Could you check a few things on this model? Use its own coordinates, in mm. Face numbers are marked on the shaded views. A direction names the side the tool comes from. Coordinates: 2 decimals unless noted, no trailing zeros. Write each loop counter-clockwise with the first axis right and the second up, starting at its lowest first coordinate (ties: lowest second). Pieces come first, ordered by that corner, then holes. Notation, with made-up numbers: (-13, 59.25) - (35, 59.25) arc R22 cw to (35, 87.25) - close; hole circle Ø11 at (9, 27.5). An arc over 180 degrees is marked (long way). Answer as a JSON object with one key per item and string values. Group by question number.
1) If we section it at C-C (z = 1): Write out the boundary of the cut face in (x, y), plus the area to 3 significant figures.
2) If we section it at B-B (x = -8.5): Write out the boundary of the cut face in (y, z), plus the area to 3 significant figures.
3) If we section it at A-A (y = 9): Write out the boundary of the cut face in (x, z).
4) We'd pull the mould along X, two halves only. Please class the marked faces 4, 5 and 6: released by +X, released by -X, zero draft, split by the parting line, or undercut.
5) If we section it at D-D (z = 9): Write out the boundary of the cut face in (x, y), plus the area to 3 significant figures.
6) On a 3-axis mill with a long thin cutter (end or side, diameter ignored), from which of +Z, -Z, +X, -X, +Y, -Y can I reach the whole of each face in a straight line? I mean the marked faces 1, 2 and 3. Say none if no direction works.
7) Please list where these lines run through material, in increasing order: line 1 along X through (y, z) = (4.75, -10.5); line 2 along Z through (x, y) = (-8, 3.75); line 3 along Y through (x, z) = (-21, 2.5).
8) Will these pins go through, and if not, where does the flat tip stop? pin 1 Ø9.5 at (x, z) = (24.5, -13.5) entering from +Y; pin 2 Ø3 at (x, y) = (8, 5.5) entering from -Z; pin 3 Ø0.5 at (x, y) = (-21, 8) entering from +Z; pin 4 Ø4 at (x, z) = (-8.5, -6) entering from +Y.
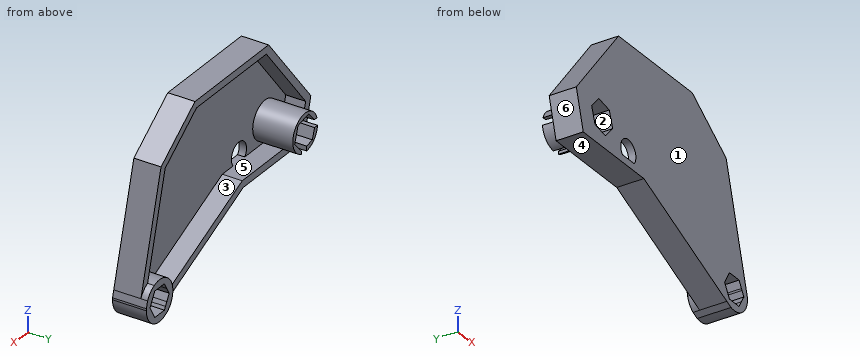
```python
from build123d import *

# Parameters (mm, degrees)
F0_R     = 3.93
F1_DEPTH = 1.5
F2_DEPTH = 5.62
F3_DEPTH = 9.8
F4_DEPTH = 7
F7_DEPTH = 3


with BuildPart() as f1:
    # F0 (on Front) → F1 (new body)
    with BuildSketch(Plane.XZ):
        with BuildLine():
            Line((-22.505389868, -2.0895681901), (-11.2077256692, -2.0895681901))
            ThreePointArc((-11.2077256692, -2.0895681901), (-9.3285928413, 1.8148319814), (-7.4494600134, -2.0895681901))
            Line((-7.4494600134, -2.0895681901), (-4.0605032691, -2.0895681901))
            Line((-4.0605032691, -2.0895681901), (20.2483866423, -12.9712812224))
            ThreePointArc((20.2483866423, -12.9712812224), (21.5778297936, -8.6925507754), (26.0093476524, -8.0317915166))
            Line((26.0093476524, -8.0317915166), (20.4338732281, 12.2993333716))
            Line((20.4338732281, 12.2993333716), (10.4662147941, 19.5698092025))
            Line((10.4662147941, 19.5698092025), (-11.712607269, 19.5698092025))
            Line((-11.712607269, 19.5698092025), (-24.1958881701, 4.0444751638))
            Line((-24.1958881701, 4.0444751638), (-22.505389868, -2.0895681901))
        make_face()
        with Locations((-17.636482101, 2.2704318099)):
            Circle(F0_R, mode=Mode.SUBTRACT)
    extrude(amount=-F1_DEPTH)

    # F0 (on Front) → F2 (join)
    with BuildSketch(Plane.XZ):
        with BuildLine():
            Line((-7.4494600134, -2.0895681901), (-9.3285928413, -2.0895681901))
            Line((-9.3285928413, -2.0895681901), (-11.2077256692, -2.0895681901))
            Line((-11.2077256692, -2.0895681901), (-22.505389868, -2.0895681901))
            Line((-22.505389868, -2.0895681901), (-24.1958881701, 4.0444751638))
            Line((-24.1958881701, 4.0444751638), (-11.712607269, 19.5698092025))
            Line((-11.712607269, 19.5698092025), (10.4662147941, 19.5698092025))
            Line((10.4662147941, 19.5698092025), (20.4338732281, 12.2993333716))
            Line((20.4338732281, 12.2993333716), (26.0093476524, -8.0317915166))
            ThreePointArc((26.0093476524, -8.0317915166), (27.2575403042, -8.8716753621), (28.1309747483, -10.096625174))
            Line((28.1309747483, -10.096625174), (21.7417066053, 13.2020214837))
            Line((21.7417066053, 13.2020214837), (10.9551470408, 21.0698092025))
            Line((10.9551470408, 21.0698092025), (-12.4312654999, 21.0698092025))
            Line((-12.4312654999, 21.0698092025), (-25.8459559813, 4.3860902027))
            Line((-25.8459559813, 4.3860902027), (-23.6479217985, -3.5895681901))
            Line((-23.6479217985, -3.5895681901), (-4.3809167168, -3.5895681901))
            Line((-4.3809167168, -3.5895681901), (21.9651791943, -15.3832229506))
            ThreePointArc((21.9651791943, -15.3832229506), (20.887904522, -14.3330472271), (20.2483866423, -12.9712812224))
            Line((20.2483866423, -12.9712812224), (-4.0605032691, -2.0895681901))
            Line((-4.0605032691, -2.0895681901), (-7.4494600134, -2.0895681901))
        make_face()
    extrude(amount=-F2_DEPTH)

    # F0 (on Front) → F3 (join)
    with BuildSketch(Plane.XZ):
        with Locations((-17.636482101, 2.2704318099)):
            Circle(F0_R)
        Polygon((-16.5711225386, -0.9650499681), (-19.9058117331, -0.2699375244), (-20.9711712955, 2.9655442536), (-18.7018416635, 5.5059135879), (-15.367152469, 4.8108011442), (-14.3017929065, 1.5753193661), align=None, mode=Mode.SUBTRACT)
    extrude(amount=-F3_DEPTH)

    # F0 (on Front) → F4 (join)
    with BuildSketch(Plane.XZ):
        with BuildLine():
            Line((22.4537352546, -13.9584908738), (20.2483866423, -12.9712812224))
            ThreePointArc((20.2483866423, -12.9712812224), (20.887904522, -14.3330472271), (21.9651791943, -15.3832229506))
            Line((21.9651791943, -15.3832229506), (23.2829635099, -15.9731203426))
            ThreePointArc((23.2829635099, -15.9731203426), (26.905846951, -15.2153095013), (28.5319774541, -11.8903641956))
            ThreePointArc((28.5319774541, -11.8903641956), (28.5271836329, -11.6894581734), (28.5128130807, -11.4890094325))
            Line((28.5128130807, -11.4890094325), (28.1309747483, -10.096625174))
            ThreePointArc((28.1309747483, -10.096625174), (27.2575403042, -8.8716753621), (26.0093476524, -8.0317915166))
            Line((26.0093476524, -8.0317915166), (26.7851210641, -10.8606711631))
            Line((26.7851210641, -10.8606711631), (27.3796146136, -11.8903641956))
            Line((27.3796146136, -11.8903641956), (26.6146255071, -13.2153641953))
            Line((26.6146255071, -13.2153641953), (25.8496364003, -14.5403641956))
            Line((25.8496364003, -14.5403641956), (24.3196581869, -14.5403641956))
            Line((24.3196581869, -14.5403641956), (22.7896799735, -14.5403641956))
            Line((22.7896799735, -14.5403641956), (22.4537352546, -13.9584908738))
        make_face()
        with BuildLine():
            ThreePointArc((26.0093476524, -8.0317915166), (21.5778297936, -8.6925507754), (20.2483866423, -12.9712812224))
            Line((20.2483866423, -12.9712812224), (22.4537352546, -13.9584908738))
            Line((22.4537352546, -13.9584908738), (22.024690908, -13.2153642668))
            Line((22.024690908, -13.2153642668), (21.2597017602, -11.8903641956))
            Line((21.2597017602, -11.8903641956), (22.0246909248, -10.5653640952))
            Line((22.0246909248, -10.5653640952), (22.7896799735, -9.2403641956))
            Line((22.7896799735, -9.2403641956), (24.3196581869, -9.2403641956))
            Line((24.3196581869, -9.2403641956), (25.8496364003, -9.2403641956))
            Line((25.8496364003, -9.2403641956), (26.6146254836, -10.5653641553))
            Line((26.6146254836, -10.5653641553), (26.7851210641, -10.8606711631))
            Line((26.7851210641, -10.8606711631), (26.0093476524, -8.0317915166))
        make_face()
    extrude(amount=-F4_DEPTH)

    # F6 (on face) → F7 (cut)
    with BuildSketch(Plane(origin=(0, 9.8, 0), x_dir=(-1, 0, 0), z_dir=(0, 1, 0))):
        with BuildLine():
            ThreePointArc((16.5027278304, -1.4924794638), (17.2955343411, -1.6447507689), (18.1027278304, -1.6318130466))
            Line((18.1027278304, -1.6318130466), (18.1027278304, -0.6457884612))
            Line((18.1027278304, -0.6457884612), (16.5711225386, -0.9650499681))
            Line((16.5711225386, -0.9650499681), (16.5027278304, -0.8884864682))
            Line((16.5027278304, -0.8884864682), (16.5027278304, -1.4924794638))
        make_face()
        with BuildLine():
            Line((20.9711712955, 2.9655442536), (20.60459144, 1.852246467))
            Line((20.60459144, 1.852246467), (21.544169527, 1.852246467))
            ThreePointArc((21.544169527, 1.852246467), (21.5608999932, 2.0610417242), (21.566482101, 2.2704318099))
            ThreePointArc((21.566482101, 2.2704318099), (21.520739578, 2.8682978924), (21.3845768325, 3.452246467))
            Line((21.3845768325, 3.452246467), (20.5363968161, 3.452246467))
            Line((20.5363968161, 3.452246467), (20.9711712955, 2.9655442536))
        make_face()
    extrude(amount=-F7_DEPTH, mode=Mode.SUBTRACT)


solid = f1.part
```
Here are the results:
{
 "1": {"outline": "(-24.91, 0) - (-20.32, 0) - (-20.32, 9.8) - (-21.36, 9.8) - (-21.36, 1.5) - (-23.36, 1.5) - (-23.36, 5.62) - (-24.91, 5.62) - close; (-14.82, 0) - (-11.13, 0) - (-11.13, 1.5) - (-13.92, 1.5) - (-13.92, 9.8) - (-14.82, 9.8) - close; (-7.52, 0) - (25.09, 0) - (25.09, 5.62) - (23.53, 5.62) - (23.53, 1.5) - (-7.52, 1.5) - close", "area": "90.2 mm²"},
 "2": {"outline": "(0, -3.59) - (5.62, -3.59) - (5.62, -2.09) - (0, -2.09) - close; (0, 1.67) - (1.5, 1.67) - (1.5, 19.57) - (5.62, 19.57) - (5.62, 21.07) - (0, 21.07) - close", "area": "43.7 mm²"},
 "3": {"outline": "(-21.54, 1.85) arc R3.93 ccw to (-18.1, -1.63) - (-18.1, -0.65) - (-19.91, -0.27) - (-20.6, 1.85) - close; (-21.38, 3.45) - (-20.54, 3.45) - (-18.7, 5.51) - (-15.37, 4.81) - (-14.3, 1.58) - (-16.5, -0.89) - (-16.5, -1.49) arc R3.93 ccw (long way) to start"},
 "4": {"face 4": "zero draft", "face 5": "undercut", "face 6": "released by -X"},
 "5": {"outline": "(-22.14, 0) - (22.89, 0) - (22.89, 5.62) - (21.34, 5.62) - (21.34, 1.5) - (-20.21, 1.5) - (-20.21, 5.62) - (-22.14, 5.62) - close", "area": "81.9 mm²"},
 "6": {"face 1": "+Z, -Z, +X, -X, -Y", "face 2": "+Y, -Y", "face 3": "+Y"},
 "7": {"line 1": "x = 11.06 to 14.73, 20.34 to 22.06, 26.58 to 28.24", "line 2": "z = -3.59 to -2.09, 19.57 to 21.07", "line 3": "y = 0 to 6.8"},
 "8": {"pin 1": "stops at y = 7", "pin 2": "stops at z = -9.8", "pin 3": "stops at z = 4.67", "pin 4": "passes through"}
}
